The model under review builds one solid part; all positions refer to its coordinate system, in mm. A direction names the side the tool comes from. Give positions to 0.01 mm unless a question says otherwise; leave off trailing zeros. Write each loop counter-clockwise with the first axis right and the second up, starting at its lowest first coordinate (ties: lowest second). Pieces come first, ordered by that corner, then holes. Notation, with made-up numbers: M 87,22 L 130,22 A6 cw 130,26 Z; hole C 82.25,83.25 d2. An arc over 180 degrees is marked long. Write item = value, one per line. Start each with the question number.
```python
from build123d import *

# Parameters (mm, degrees)
CROQUIS1_R                                           = 5
SALIENTE_EXTRUIR1_DEPTH                              = 10
CROQUIS2_R                                           = 32.7
SALIENTE_EXTRUIR2_DEPTH                              = 53.5
CROQUIS3_R                                           = 21.5
CORTAR_EXTRUIR2_DEPTH                                = 55
REFRENTADO_PARA_TORNILLO_CON_CABEZA_TRON_D           = 3.4
REFRENTADO_PARA_TORNILLO_CON_CABEZA_TRON_CBORE_D     = 7
REFRENTADO_PARA_TORNILLO_CON_CABEZA_TRON_CBORE_DEPTH = 2.4
TALADRO_DE_MARGEN_PARA_M31_D                         = 3.4
TALADRO_DE_MARGEN_PARA_M31_DEPTH                     = 16
TALADRO_DE_MARGEN_PARA_M31_TIP                       = 1.021463052
CORTAR_EXTRUIR3_DEPTH                                = 5
CROQUIS11_R                                          = 42.5
SALIENTE_EXTRUIR3_DEPTH                              = 7.5
TALADRO_DE_MARGEN_PARA_M32_D                         = 3.4
TALADRO_DE_MARGEN_PARA_M32_DEPTH                     = 16
TALADRO_DE_MARGEN_PARA_M32_TIP                       = 1.021463052
REFRENTADO_PARA_TORNILLO_CON_CABEZA_2_D              = 3.4
REFRENTADO_PARA_TORNILLO_CON_CABEZA_2_CBORE_D        = 7
REFRENTADO_PARA_TORNILLO_CON_CABEZA_2_CBORE_DEPTH    = 2.4


with BuildPart() as part:
    # Croquis1 → Saliente-Extruir1 (new body)
    with BuildSketch(Plane(origin=(0, 0, 0), x_dir=(0, 0, -1), z_dir=(1, 0, 0))):
        Polygon((-21.75, -17.75), (-21.75, 17.75), (-17.75, 21.75), (17.75, 21.75), (21.75, 17.75), (21.75, -17.75), (17.75, -21.75), (-17.75, -21.75), align=None)
        Circle(CROQUIS1_R, mode=Mode.SUBTRACT)
    extrude(amount=SALIENTE_EXTRUIR1_DEPTH)

    # Croquis2 → Saliente-Extruir2 (add)
    with BuildSketch(Plane.ZY):
        Circle(CROQUIS2_R)
    extrude(amount=SALIENTE_EXTRUIR2_DEPTH)

    # Croquis3 → Cortar-Extruir2 (cut)
    with BuildSketch(Plane.ZY.offset(53.5)):
        Circle(CROQUIS3_R)
    extrude(amount=-CORTAR_EXTRUIR2_DEPTH, mode=Mode.SUBTRACT)

    # Refrentado para tornillo con cabeza tron (through all)
    with Locations(Plane(origin=(10, 0, 0), x_dir=(0, 0, -1), z_dir=(1, 0, 0))):
        with Locations((-8.838834765, 8.838834765), (8.838834765, 8.838834765), (8.838834765, -8.838834765), (-8.838834765, -8.838834765)):
            CounterBoreHole(REFRENTADO_PARA_TORNILLO_CON_CABEZA_TRON_D / 2, REFRENTADO_PARA_TORNILLO_CON_CABEZA_TRON_CBORE_D / 2, REFRENTADO_PARA_TORNILLO_CON_CABEZA_TRON_CBORE_DEPTH)

    # Taladro de margen para M31
    with Locations(Plane(origin=(10, 0, 0), x_dir=(0, 0, -1), z_dir=(1, 0, 0))):
        with Locations((15.5, 15.5), (15.5, -15.5), (-15.5, -15.5), (-15.5, 15.5)):
            Hole(TALADRO_DE_MARGEN_PARA_M31_D / 2, depth=TALADRO_DE_MARGEN_PARA_M31_DEPTH)
            with Locations((0, 0, -(TALADRO_DE_MARGEN_PARA_M31_DEPTH + TALADRO_DE_MARGEN_PARA_M31_TIP / 2))):  # 118° drill point
                Cone(0, TALADRO_DE_MARGEN_PARA_M31_D / 2, TALADRO_DE_MARGEN_PARA_M31_TIP, mode=Mode.SUBTRACT)

    # Croquis10 → Cortar-Extruir3 (cut)
    with BuildSketch(Plane.ZY.offset(-1.5)):
        Polygon((-13.251400436, 13.251400436), (-12.428355872, 16.323044563), (-14.676955437, 18.571644128), (-17.748599564, 17.748599564), (-18.571644128, 14.676955437), (-16.323044563, 12.428355872), align=None)
        Polygon((18.571644128, 14.676955437), (17.748599564, 17.748599564), (14.676955437, 18.571644128), (12.428355872, 16.323044563), (13.251400436, 13.251400436), (16.323044563, 12.428355872), align=None)
        Polygon((14.676955437, -18.571644128), (17.748599564, -17.748599564), (18.571644128, -14.676955437), (16.323044563, -12.428355872), (13.251400436, -13.251400436), (12.428355872, -16.323044563), align=None)
        Polygon((-18.571644128, -14.676955437), (-17.748599564, -17.748599564), (-14.676955437, -18.571644128), (-12.428355872, -16.323044563), (-13.251400436, -13.251400436), (-16.323044563, -12.428355872), align=None)
    extrude(amount=CORTAR_EXTRUIR3_DEPTH, mode=Mode.SUBTRACT)

    # Croquis11 → Saliente-Extruir3 (add)
    with BuildSketch(Plane.ZY.offset(53.5)):
        Circle(CROQUIS11_R)
        Polygon((-21.5, -17.75), (-21.5, 17.75), (-17.75, 21.5), (17.75, 21.5), (21.5, 17.75), (21.5, -17.75), (17.75, -21.5), (-17.75, -21.5), align=None, mode=Mode.SUBTRACT)
    extrude(amount=SALIENTE_EXTRUIR3_DEPTH)

    # Taladro de margen para M32
    with Locations(Plane.ZY.offset(53.5)):
        with Locations((-17.075, 17.075), (17.075, 17.075), (17.075, -17.075), (-17.075, -17.075)):
            Hole(TALADRO_DE_MARGEN_PARA_M32_D / 2, depth=TALADRO_DE_MARGEN_PARA_M32_DEPTH)
            with Locations((0, 0, -(TALADRO_DE_MARGEN_PARA_M32_DEPTH + TALADRO_DE_MARGEN_PARA_M32_TIP / 2))):  # 118° drill point
                Cone(0, TALADRO_DE_MARGEN_PARA_M32_D / 2, TALADRO_DE_MARGEN_PARA_M32_TIP, mode=Mode.SUBTRACT)

    # Refrentado para tornillo con cabeza  2 (through all)
    with Locations(Plane(origin=(-53.5, 0, 0), x_dir=(0, 0, -1), z_dir=(1, 0, 0))):
        with Locations((0, 37.6), (32.562555182, 18.8), (32.562555182, -18.8), (0, -37.6), (-32.562555182, -18.8), (-32.562555182, 18.8)):
            CounterBoreHole(REFRENTADO_PARA_TORNILLO_CON_CABEZA_2_D / 2, REFRENTADO_PARA_TORNILLO_CON_CABEZA_2_CBORE_D / 2, REFRENTADO_PARA_TORNILLO_CON_CABEZA_2_CBORE_DEPTH)


solid = part.part
```
Item 1: To check wall thickness, follow probe 1 along Z at (x, y) = (7.25, -15.5); probe 2 along Y at (x, z) = (-50, -18.5); probe 3 along Z at (x, y) = (-59, -18). State the ranges of each line that lie inside material, in increasing order. Write a range as [from, to].
Item 2: For faces 3 (the cylindrical face through (-58.49, 38.75, -1.25)), 4 (the flat face through (-0.965, -16.191, -18.166)), 5 (the flat face through (-57.2, -19.6, 19.65)), 6 (the cylindrical face through (5.7, 14, -14.7)), list the 3-axis set-ups (+Z, -Z, +X, -X, +Y, -Y) from which the entire face can be reached by the end or side of a thin tool; tool diameter is ignored.
Item 3: We need section A-A, the plane x = -26. Write out the cut boundary in (y, z).
Item 4: Clearance check with flat-ended pins moving along their axes: P1, Ø2.5, axis at y = 37.6, z = 0, coming from the -X side; P2, Ø3.5, axis at y = -18, z = -32, coming from the +X side; P3, Ø1, axis at x = -49.5, y = -13, coming from the +Z side; P4, Ø1, axis at x = -40, y = 17, coming from the -Z side. State where each tip first meets the part, or that it passes through.
Item 5: We need section C-C, the plane y = 27.5. Write out the cut boundary in (x, z).
Item 6: We need section B-B, the plane x = -48.5. Write out the cut boundary in (y, z) (3 decimals).
Item 7: The part is to be moulded in two halves that separate along Y. For faces 1 (the flat face through (-53.5, 10, -32)), 2 (the flat face through (-55.9, -17, -33)), say which applies: released by +Y, released by -Y, zero draft, split by the parting line, or undercut.
Worked out:
q1.probe_1 = [-21.75, -17.2], [-13.8, 13.8], [17.2, 21.75]
q1.probe_2 = [-26.96, -18], [-16.15, -10.95], [10.95, 16.15], [18, 26.96]
q1.probe_3 = [-38.5, -34.06], [-31.06, -21.25], [21.25, 31.06], [34.06, 38.5]
q2.face_3 = +X, -X
q2.face_4 = none
q2.face_5 = -X
q2.face_6 = +X
q3.outline = C 0,0 d65.4; hole C 0,0 d43
q4.P1 = through
q4.P2 = -55.9
q4.P3 = 30.22
q4.P4 = -28.23
q5.outline = M -61,-32.4 L -53.5,-32.4 L -53.5,-17.69 L 0,-17.69 L 0,17.69 L -53.5,17.69 L -53.5,32.4 L -61,32.4 Z
q6.outline = C 0,0 d65.4; hole C 0,0 d43; hole C -17.075,-17.075 d3.4; hole C -17.075,17.075 d3.4; hole C 17.075,-17.075 d3.4; hole C 17.075,17.075 d3.4
q7.face_1 = zero draft
q7.face_2 = undercut
